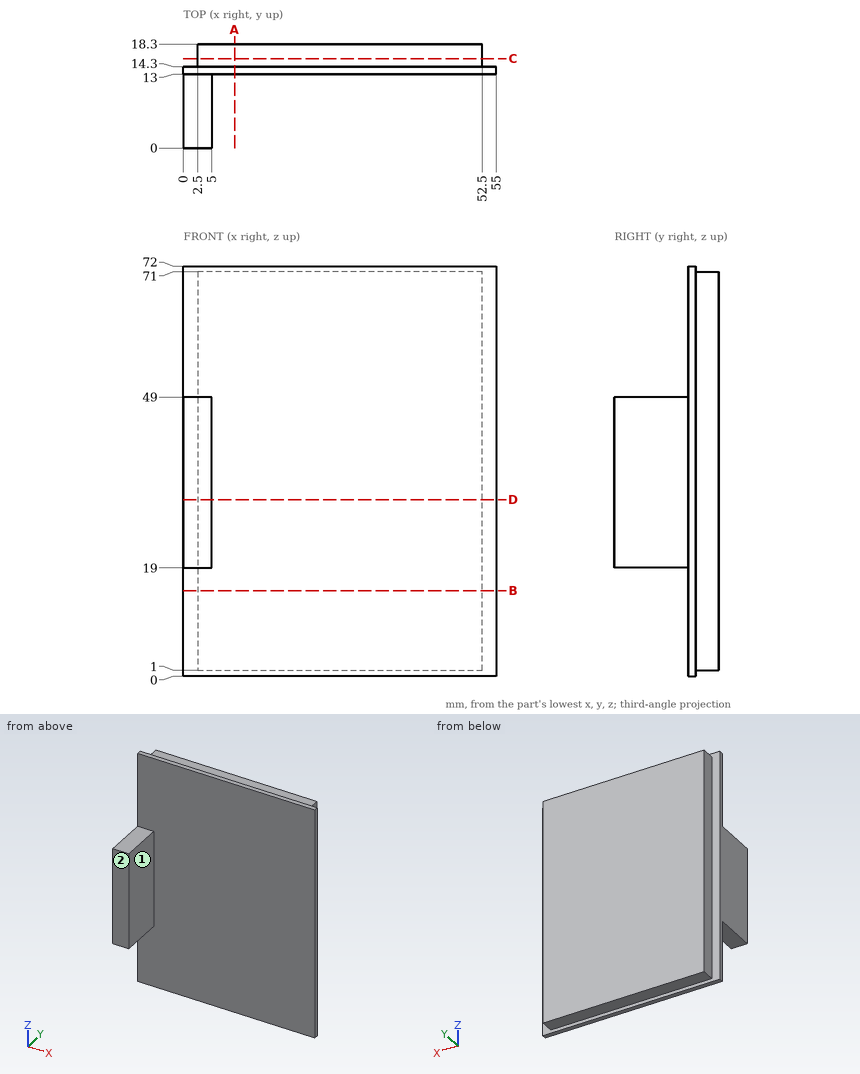
Can you work these out from the drawing? Everything is in mm from the part's minimum corner. A direction names the side the tool comes from. Give positions to 0.01 mm unless a question says otherwise; leave off trailing zeros. Order: outer loops, then holes, each group sorted by start corner. A loop starts at its lowest first (then second) coordinate and runs counter-clockwise, first axis right, second up. Notation, with made-up numbers: M -1.5,6 L 50.5,6 A30 ccw 50.5,30 Z; hole C -5,63.5 d8. An arc over 180 degrees is marked long. Use a Markdown table: item, result. Add a question column.
Item 1: Suppose I cut it at B-B (z = 15). List the corners of the cut face in (x, y) for me.
Item 2: Will these pins go through, and if not, where does the flat tip stop? pin 1 (4.5 mm diameter, centred on y = 17, z = 22.5, fed in from -X); pin 2 (3 mm diameter, centred on x = 21.5, y = 16.5, fed in from -Z); pin 3 (2 mm diameter, centred on x = 16.5, y = 16, fed in from +Z).
Item 3: Suppose I cut it at C-C (y = 15.75). List the corners of the cut face in (x, z) for me, then the cut area to 3 significant figures.
Item 4: For the marked faces 1 and 2, which set-ups out of +Z, -Z, +X, -X, +Y, -Y let a thin tool reach every point of the face, with its end or its side?
Item 5: Suppose I cut it at A-A (x = 9). List the corners of the cut face in (y, z) for me, then the cut area to 3 significant figures.
Item 6: Suppose I cut it at D-D (z = 31). List the corners of the cut face in (x, y) for me, then the cut area to 4 significant figures.
Item 7: If I drill on L1, parallel to X at y = 15.75, z = 68.5; L2, parallel to Y at x = 46, z = 53.5; L3, parallel to Z at x = 3.5, y = 17.5, over which ranges is the centre line in solid material (lowest first)? Write a range as [from, to].
Answer sheet:
| question | item | result |
|---|---|---|
| 1 | outline | M 0,13 L 55,13 L 55,14.3 L 52.5,14.3 L 52.5,18.3 L 2.5,18.3 L 2.5,14.3 L 0,14.3 Z |
| 2 | pin 1 | stops at x = 2.5 |
| 2 | pin 2 | stops at z = 1 |
| 2 | pin 3 | stops at z = 71 |
| 3 | outline | M 2.5,1 L 52.5,1 L 52.5,71 L 2.5,71 Z |
| 3 | area | 3,500 mm² |
| 4 | face 1 | +Z, -Z, +X, -Y |
| 4 | face 2 | +Z, -Z, +X, -X, -Y |
| 5 | outline | M 13,0 L 14.3,0 L 14.3,1 L 18.3,1 L 18.3,71 L 14.3,71 L 14.3,72 L 13,72 Z |
| 5 | area | 374 mm² |
| 6 | outline | M 0,0 L 5,0 L 5,13 L 55,13 L 55,14.3 L 52.5,14.3 L 52.5,18.3 L 2.5,18.3 L 2.5,14.3 L 0,14.3 Z |
| 6 | area | 336.5 mm² |
| 7 | L1 | x = [2.5, 52.5] |
| 7 | L2 | y = [13, 18.3] |
| 7 | L3 | z = [1, 71] |
